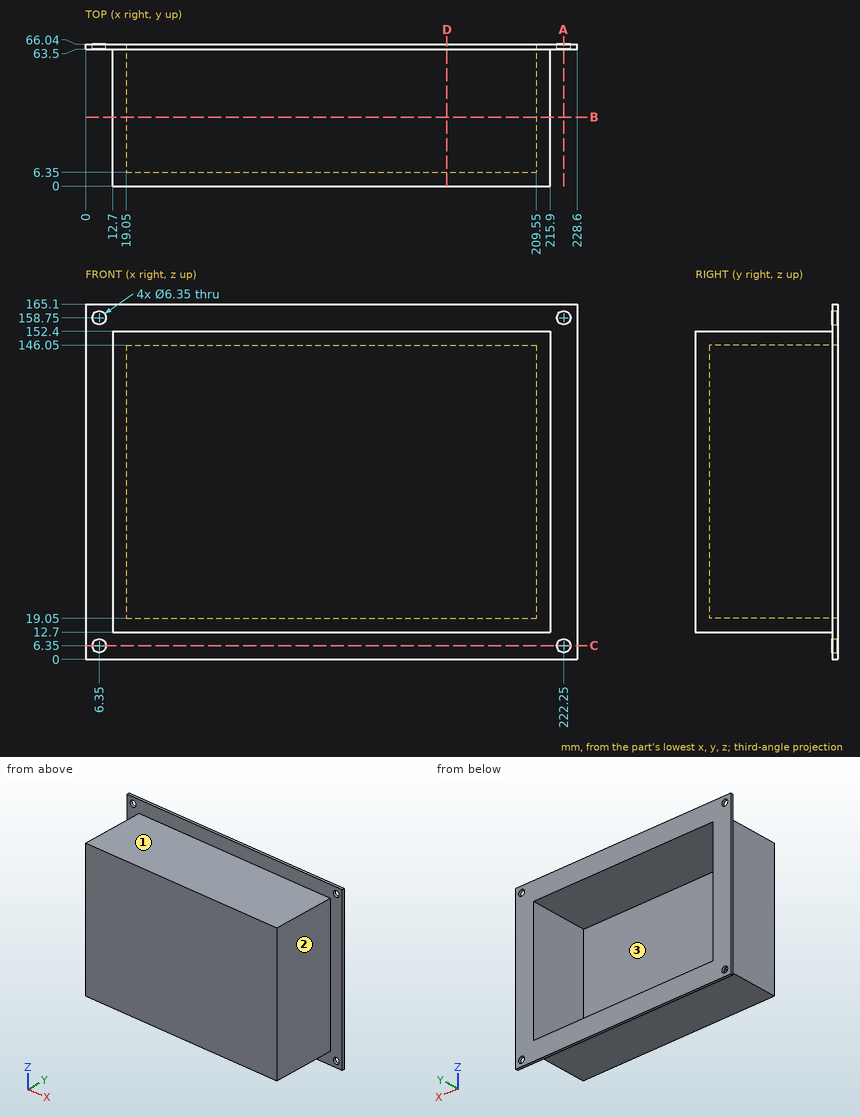
Here's the drawing with two shaded views (mm, measured from the low corner). I have some questions. A direction names the side the tool comes from. Give positions to 0.01 mm unless a question says otherwise; leave off trailing zeros. Loops run counter-clockwise (first coordinate to the right, second up) from the corner with the lowest first, then second, coordinate; pieces in that order, holes last. Notation, with made-up numbers: (49, 15.25) - (76, 15.25) arc R9 ccw to (76, 23.25) - close; hole circle Ø6 at (28.25, -23). An arc over 180 degrees is marked (long way). Return JSON: item names as keys, results as strings.
1. I want a section at B-B on y = 32. Please give me the cut outline in (x, z), and give its area (3 significant figures).
Output values:
{"outline": "(12.7, 12.7) - (215.9, 12.7) - (215.9, 152.4) - (12.7, 152.4) - close; hole (19.05, 19.05) - (209.55, 19.05) - (209.55, 146.05) - (19.05, 146.05) - close", "area": "4,190 mm²"}
2. If I drill on line 1 (X direction, y = 65.15, z = 158.75) (3 decimals); line 2 (Z direction, x = 222.25, y = 64.8) (3 decimals); line 3 (Z direction, x = 131.5, y = 14.5), over which ranges is the centre line in solid material (lowest first)?
Output values:
{"line 1": "x = 0 to 3.175, 9.525 to 219.075, 225.425 to 228.6", "line 2": "z = 0 to 3.175, 9.525 to 155.575, 161.925 to 165.1", "line 3": "z = 12.7 to 19.05, 146.05 to 152.4"}
3. I want a section at C-C on z = 6.35. Please give me the cut outline in (x, y) (3 decimals).
Output values:
{"outline": "(0, 63.5) - (3.175, 63.5) - (3.175, 66.04) - (0, 66.04) - close; (9.525, 63.5) - (219.075, 63.5) - (219.075, 66.04) - (9.525, 66.04) - close; (225.425, 63.5) - (228.6, 63.5) - (228.6, 66.04) - (225.425, 66.04) - close"}
4. For the marked faces 1, 2 and 3, which set-ups out of +Z, -Z, +X, -X, +Y, -Y let a thin tool reach every point of the face, with its end or its side?
Output values:
{"face 1": "+Z, +X, -X, -Y", "face 2": "+Z, -Z, +X, -Y", "face 3": "+Y"}
5. I want a section at A-A on x = 222.25. Please give me the cut outline in (y, z) (3 decimals).
Output values:
{"outline": "(63.5, 0) - (66.04, 0) - (66.04, 3.175) - (63.5, 3.175) - close; (63.5, 9.525) - (66.04, 9.525) - (66.04, 155.575) - (63.5, 155.575) - close; (63.5, 161.925) - (66.04, 161.925) - (66.04, 165.1) - (63.5, 165.1) - close"}
6. I'm going to push flat-ended pins straight in: pin 1 Ø8 at (y, z) = (51, 74.5) entering from +X; pin 2 Ø12 at (x, y) = (78, 49) entering from -Z; pin 3 Ø12 at (x, y) = (83, 15.5) entering from +Z. Where does each tip first touch, or does it pass through?
Output values:
{"pin 1": "stops at x = 215.9", "pin 2": "stops at z = 12.7", "pin 3": "stops at z = 152.4"}
7. I want a section at D-D on x = 168. Please give me the cut outline in (y, z), and give its area (3 significant figures).
Output values:
{"outline": "(0, 12.7) - (63.5, 12.7) - (63.5, 0) - (66.04, 0) - (66.04, 19.05) - (6.35, 19.05) - (6.35, 146.05) - (66.04, 146.05) - (66.04, 165.1) - (63.5, 165.1) - (63.5, 152.4) - (0, 152.4) - close", "area": "1,710 mm²"}
